```python
from build123d import *

# Parameters (mm, degrees)
CROQUIS1_R              = 4.5
SALIENTE_EXTRUIR1_DEPTH = 9.5
CORTAR_EXTRUIR1_START   = -8.5
CROQUIS2_R              = 4.5
CROQUIS2_R_2            = 3.75
CORTAR_EXTRUIR1_DEPTH   = 8.5
REDONDEO1_R             = 0.5


with BuildPart() as part:
    # Croquis1 → Saliente-Extruir1 (new body)
    with BuildSketch(Plane(origin=(0, 0, 0), x_dir=(1, 0, 0), z_dir=(0, 1, 0))):
        with Locations(Location((0, 0, 0), (0, 0, 270))):
            Circle(CROQUIS1_R)
    extrude(amount=SALIENTE_EXTRUIR1_DEPTH)

    # Croquis2 → Cortar-Extruir1 (cut)
    with BuildSketch(Plane(origin=(0, 9.5, 0), x_dir=(1, 0, 0), z_dir=(0, 1, 0)).offset(CORTAR_EXTRUIR1_START)):
        with Locations(Location((0, 0, 0), (0, 0, 270))):
            Circle(CROQUIS2_R)
        with Locations(Location((0, 0, 0), (0, 0, 270))):
            Circle(CROQUIS2_R_2, mode=Mode.SUBTRACT)
    extrude(amount=CORTAR_EXTRUIR1_DEPTH, mode=Mode.SUBTRACT)

    # Redondeo1
    redondeo1_edges = [part.edges().sort_by_distance(p)[0] for p in [
        (0, 9.5, -3.75),
    ]]
    fillet(redondeo1_edges, radius=REDONDEO1_R)


solid = part.part
```
Geometry: final body of the model. Coordinates: model frame, mm. A direction names the side the tool comes from. Round coordinates to 2 decimals unless told otherwise and drop trailing zeros. Order: outer loops, then holes, each group sorted by start corner. A loop starts at its lowest first (then second) coordinate and runs counter-clockwise, first axis right, second up. Notation, with made-up numbers: (25, -28.75) -> (73, -28.75) arc R24 ccw to (73, 8.25) -> close; hole circle Ø8 at (30.25, 44). An arc over 180 degrees is marked (long way). Use CSV: the item, a comma, the result in double quotes. Start each with the question number.
1) Set-up query: faces 1 (the face through (1.352, 0.493, 4.292)), 2 (the face through (4, 1, -1)). Return all of +Z, -Z, +X, -X, +Y, -Y with unobstructed straight access to the full face (end or side cutting, diameter ignored); none if empty.
2) Section B-B (z = 0). Return the cut outline in (x, y), and give its area (3 significant figures).
3) First-contact query: pin 1 Ø2 at (y, z) = (4, 2.5) entering from -X; pin 2 Ø1 at (y, z) = (4.5, -3.5) entering from -X. Flat tips, straight axial feed; report the tip coordinate or a pass-through.
4) Material intervals for line 1 along Y through (x, z) = (-3, 3); line 2 along X through (y, z) = (2.25, 2.75); line 3 along X through (y, z) = (4.5, -3.25), sorted ascending. Write a range as from..to.
5) Section D-D (x = -4). Return the cut outline in (y, z), and give its area (3 significant figures).
6) Section C-C (y = 5). Return the cut outline in (x, z).
7) Section A-A (x = 0). Return the cut outline in (y, z).
Returned:
1,face 1,"+Y, -Y"
1,face 2,"+Y"
2,outline,"(-4.5, 0) -> (4.5, 0) -> (4.5, 1) -> (3.75, 1) -> (3.75, 9) arc R0.5 ccw to (3.25, 9.5) -> (-3.25, 9.5) arc R0.5 ccw to (-3.75, 9) -> (-3.75, 1) -> (-4.5, 1) -> close"
2,area,"72.6 mm²"
3,pin 1,"stops at x = -3.44"
3,pin 2,"stops at x = -2.25"
4,line 1,"y = 0..1"
4,line 2,"x = -2.55..2.55"
4,line 3,"x = -1.87..1.87"
5,outline,"(0, -2.06) -> (1, -2.06) -> (1, 2.06) -> (0, 2.06) -> close"
5,area,"4.12 mm²"
6,outline,"circle Ø7.5 at (0, 0)"
7,outline,"(0, -4.5) -> (1, -4.5) -> (1, -3.75) -> (9, -3.75) arc R0.5 ccw to (9.5, -3.25) -> (9.5, 3.25) arc R0.5 ccw to (9, 3.75) -> (1, 3.75) -> (1, 4.5) -> (0, 4.5) -> close"
